Source: CAD feature listing. Evaluate the final solid. Frame: model axes, mm. Face numbers are marked on the shaded views. A direction names the side the tool comes from. Round coordinates to 2 decimals unless told otherwise and drop trailing zeros. Write each loop counter-clockwise with the first axis right and the second up, starting at its lowest first coordinate (ties: lowest second). Pieces come first, ordered by that corner, then holes. Notation, with made-up numbers: M 12.5,66.25 L 61.5,66.25 A8 cw 61.5,77.25 Z; hole C 82,78.5 d11. An arc over 180 degrees is marked long. Answer in a Markdown table with one row per item.
from build123d import *

# Parameters (mm, degrees)
F1_DEPTH = 25.4
F3_DEPTH = 12.7
F5_DEPTH = 12.7
F7_DEPTH = 25.4
F8_R     = 4.9638904574
F9_DEPTH = 25.4


with BuildPart() as f1:
    # F0 (on Front) → F1 (new body)
    with BuildSketch(Plane.XZ):
        Polygon((-69.85, 38.1), (-69.85, 0), (0, 0), (0, 12.7), (-50.8, 12.7), (-50.8, 38.1), align=None)
    extrude(amount=F1_DEPTH)

    # F2 (on face) → F3 (cut)
    with BuildSketch(Plane.XY.offset(12.7)):
        with BuildLine():
            ThreePointArc((-12.7, 0), (-4.1664394472, -4.1664394472), (0, -12.7))
            Line((0, -12.7), (0, 0))
            Line((0, 0), (-12.7, 0))
        make_face()
        with BuildLine():
            Line((0, -25.4), (0, -12.7))
            ThreePointArc((0, -12.7), (-4.1912343362, -21.2087656638), (-12.7, -25.4))
            Line((-12.7, -25.4), (0, -25.4))
        make_face()
    extrude(amount=-F3_DEPTH, mode=Mode.SUBTRACT)

    # F4 (on face) → F5 (cut)
    with BuildSketch(Plane.XY.offset(12.7)):
        with BuildLine():
            ThreePointArc((-38.0139607827, -19.3930226044), (-33.5795548322, -17.5032103821), (-31.75, -13.0436055246))
            ThreePointArc((-31.75, -13.0436055246), (-33.6098719395, -8.5534774641), (-38.1, -6.6936055246))
            ThreePointArc((-38.1, -6.6936055246), (-44.4498542683, -13.0866261206), (-38.0139607827, -19.3930226044))
        make_face()
        with BuildLine():
            ThreePointArc((-38.1, -6.6936055246), (-33.6098719395, -8.5534774641), (-31.75, -13.0436055246))
            ThreePointArc((-31.75, -13.0436055246), (-33.5795548322, -17.5032103821), (-38.0139607827, -19.3930226044))
            Line((-38.0139607827, -19.3930226044), (-12.7000078464, -19.05))
            ThreePointArc((-12.7000078464, -19.05), (-19.049854295, -12.7430166511), (-12.7860391738, -6.3505829196))
            Line((-12.7860391738, -6.3505829196), (-38.1, -6.6936055246))
        make_face()
        with BuildLine():
            ThreePointArc((-6.35, -12.7), (-8.240395127, -8.1795548475), (-12.7860391738, -6.3505829196))
            ThreePointArc((-12.7860391738, -6.3505829196), (-19.049854295, -12.7430166511), (-12.7000078464, -19.05))
            Line((-12.7000078464, -19.05), (-12.5279294485, -19.0476682117))
            ThreePointArc((-12.5279294485, -19.0476682117), (-8.1494424516, -17.1288741232), (-6.35, -12.7))
        make_face()
    extrude(amount=-F5_DEPTH, mode=Mode.SUBTRACT)

    # F6 (on face) → F7 (cut)
    with BuildSketch(Plane.XZ.offset(25.4)):
        with BuildLine():
            Line((-69.85, 38.1), (-69.85, 29.6156106257))
            ThreePointArc((-69.85, 29.6156106257), (-67.6293367073, 35.171111242), (-62.4123890172, 38.1))
            Line((-62.4123890172, 38.1), (-69.85, 38.1))
        make_face()
        with BuildLine():
            Line((-50.8, 38.1), (-56.0623890172, 38.1))
            ThreePointArc((-56.0623890172, 38.1), (-52.2149677191, 34.3977887072), (-50.8, 29.2493049055))
            Line((-50.8, 29.2493049055), (-50.8, 38.1))
        make_face()
    extrude(amount=-F7_DEPTH, mode=Mode.SUBTRACT)

    # F8 (on face) → F9 (cut)
    with BuildSketch(Plane.XZ.offset(25.4)):
        with Locations((-60.8740881639, 29.2493049055)):
            Circle(F8_R)
    extrude(amount=-F9_DEPTH, mode=Mode.SUBTRACT)


solid = f1.part
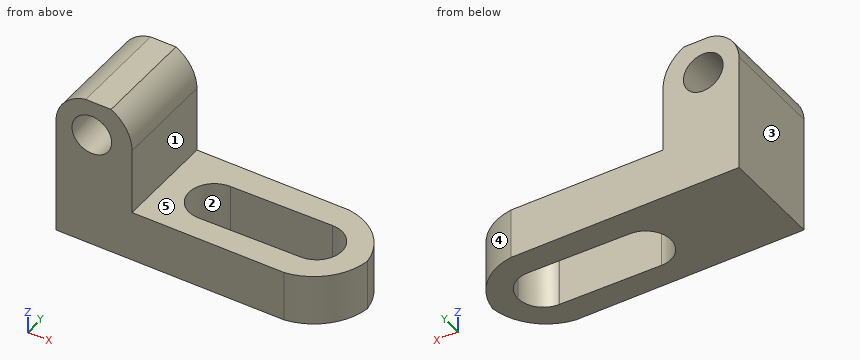
Q1. Section B-B (x = -27). Return loops of the section in (y, z), and give its area (3 significant figures).
Solutions:
| item | result |
|---|---|
| outline | M -25.4,0 L -19.24,0 L -19.24,12.7 L -25.4,12.7 Z; M -6.54,0 L 0,0 L 0,12.7 L -6.54,12.7 Z |
| area | 161 mm2 |
Q2. Pull-direction query (X, two-part tool) for the marked faces 1, 2 and 3; classes: pulls with the +X half, pulls with the -X half, needs draft (parallel to the pull), parting line crosses it, or undercut.
Solutions:
| item | result |
|---|---|
| face 1 | pulls with the +X half |
| face 2 | undercut |
| face 3 | pulls with the -X half |
Q3. Contact query for flat-ended pins moving along their axis: pin 1 Ø4 at (x, y) = (-24, -10) entering from +Z; pin 2 Ø1 at (y, z) = (-3.5, 32.5) entering from +X; pin 3 Ø4 at (y, z) = (-6, 10.5) entering from +X; pin 4 Ø8.5 at (y, z) = (-9.5, 22) entering from +X. Output: stop coordinate, or through.
Solutions:
| item | result |
|---|---|
| pin 1 | passes through |
| pin 2 | stops at x = -51.18 |
| pin 3 | stops at x = -1.41 |
| pin 4 | stops at x = -50.8 |
Q4. Section A-A (y = -10.5). Return loops of the section in (x, z).
Solutions:
| item | result |
|---|---|
| outline | M -69.85,0 L -43.92,0 L -43.92,12.7 L -50.8,12.7 L -50.8,29.25 A10.07 ccw -56.06,38.1 L -62.41,38.1 A8.98 ccw -69.85,29.62 Z; M -6.74,0 L -0.45,0 L -0.45,12.7 L -6.74,12.7 Z; hole C -60.87,29.25 d9.93 |
Q5. Section D-D (y = -7.5). Return loops of the section in (x, z).
Solutions:
| item | result |
|---|---|
| outline | M -69.85,0 L -41.2,0 L -41.2,12.7 L -50.8,12.7 L -50.8,29.25 A10.07 ccw -56.06,38.1 L -62.41,38.1 A8.98 ccw -69.85,29.62 Z; M -9.06,0 L -1.67,0 L -1.67,12.7 L -9.06,12.7 Z; hole C -60.87,29.25 d9.93 |
Q6. Access query for the marked faces 4 and 5. Directions: +Z, -Z, +X, -X, +Y, -Y. A direction counts if a zero-diameter tool reaches every point of the face in a straight line with its end or side. Return the directions, or none.
Solutions:
| item | result |
|---|---|
| face 4 | +Z, -Z, +X, +Y |
| face 5 | +Z, +X, +Y, -Y |
Q7. Section C-C (z = 15.5). Return loops of the section in (x, y), and give its area (3 significant figures).
Solutions:
| item | result |
|---|---|
| outline | M -69.85,-25.4 L -50.8,-25.4 L -50.8,0 L -69.85,0 Z |
| area | 484 mm2 |
Q8. Material intervals for probe 1 along Z at (x, y) = (-43, -7.75); probe 2 along Z at (x, y) = (-60, -17.75); probe 3 along X at (y, z) = (-10.75, 5.5), sorted ascending.
Solutions:
| item | result |
|---|---|
| probe 1 | z = 0 to 12.7 |
| probe 2 | z = 0 to 24.36, 34.14 to 38.1 |
| probe 3 | x = -69.85 to -44.02, -6.66 to -0.38 |
